The listing builds one solid part. Answer for the finished solid, in the listing's coordinates (mm). Face numbers are marked on the shaded views. A direction names the side the tool comes from. Round coordinates to 2 decimals unless told otherwise and drop trailing zeros. Loops run counter-clockwise (first coordinate to the right, second up) from the corner with the lowest first, then second, coordinate; pieces in that order, holes last. Notation, with made-up numbers: (76, 29) -> (134, 29) arc R7 cw to (134, 41) -> close; hole circle Ø10 at (30, -25). An arc over 180 degrees is marked (long way). Use a Markdown table: item, result. Add a question column.
Q1. Consider line 1 (Z direction, x = 2.25, y = 5.5) (3 decimals); line 2 (Z direction, x = 20, y = -4) (3 decimals); line 3 (Y direction, x = 1.75, z = 0). Determine where each line is inside the solid, lowest interval first.
Q2. Section B-B on y = 0 is taken. Give the vertices of the cut face in (x, z) (3 decimals), then the cut area to 3 significant figures.
Q3. Section D-D on x = 18.5 is taken. Give the vertices of the cut face in (y, z) (3 decimals).
Q4. Section C-C on z = 0 is taken. Give the vertices of the cut face in (x, y), then the cut area to 3 significant figures.
Q5. Which of the six approach directions +Z, -Z, +X, -X, +Y, -Y give full straight-line access (tool end or side, diameter ignored) to the marked faces 1 and 2?
Q6. Section A-A on x = 5.25 is taken. Give the vertices of the cut face in (y, z) (3 decimals).
Q7. Given pin 1 Ø8 at (y, z) = (7.5, -8) entering from +X; pin 2 Ø2.5 at (y, z) = (2.5, -21.5) entering from +X; pin 3 Ø1.8 at (x, y) = (12.84, 5.66) entering from +Z (3 decimals), each flat-ended and moving along its own axis, determine where each tip first touches the part or whether it passes through.
Q8. For a pull along Z with two mould halves and no side action, classify the marked faces 3, 4, 5 and 6 as released by +Z, released by -Z, zero draft, split by the parting line, or undercut.
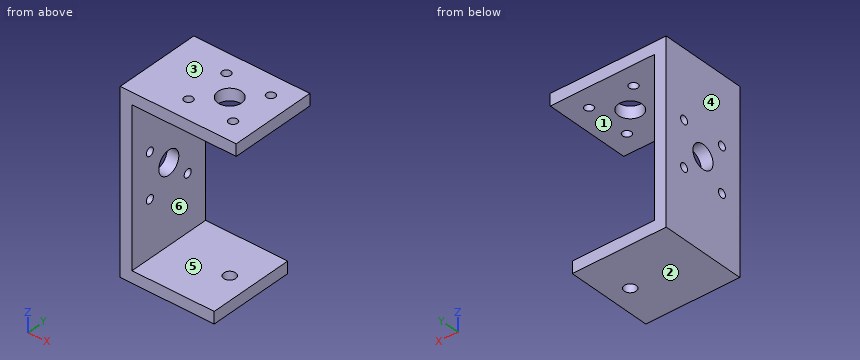
from build123d import *

# Parameters (mm, degrees)
SKETCH1_W           = 39.55
SKETCH1_H           = 22
SKETCH1_R           = 1.05
SKETCH1_R_2         = 3
BOSS_EXTRUDE1_DEPTH = 3
SKETCH1_6_W         = 3
SKETCH1_6_H         = 22
BOSS_EXTRUDE2_DEPTH = 29.5
SKETCH1_7_W         = 3
SKETCH1_7_H         = 22
BOSS_EXTRUDE3_DEPTH = 23.9
SKETCH2_R           = 3
SKETCH2_R_2         = 1.1
CUT_EXTRUDE1_DEPTH  = 3
CIRPATTERN1_COUNT   = 4
SKETCH3_R           = 1.5
CUT_EXTRUDE2_DEPTH  = 3


with BuildPart() as part:
    # Sketch1 → Boss-Extrude1 (new body)
    with BuildSketch(Plane(origin=(0, 0, 0), x_dir=(0, 0, -1), z_dir=(1, 0, 0))):
        Rectangle(SKETCH1_W, SKETCH1_H)
        with Locations((-5.656854249, -5.656854249)):
            Circle(SKETCH1_R, mode=Mode.SUBTRACT)
        with Locations((5.656854249, -5.656854249)):
            Circle(SKETCH1_R, mode=Mode.SUBTRACT)
        with Locations((-5.656854249, 5.656854249)):
            Circle(SKETCH1_R, mode=Mode.SUBTRACT)
        Circle(SKETCH1_R_2, mode=Mode.SUBTRACT)
        with Locations((5.656854249, 5.656854249)):
            Circle(SKETCH1_R, mode=Mode.SUBTRACT)
    extrude(amount=BOSS_EXTRUDE1_DEPTH)

    # Sketch1<6> → Boss-Extrude2 (add)
    with BuildSketch(Plane(origin=(0, 0, 0), x_dir=(0, 0, -1), z_dir=(1, 0, 0))):
        with Locations((-21.275, 0)):
            Rectangle(SKETCH1_6_W, SKETCH1_6_H)
    extrude(amount=BOSS_EXTRUDE2_DEPTH)

    # Sketch1<7> → Boss-Extrude3 (add)
    with BuildSketch(Plane(origin=(0, 0, 0), x_dir=(0, 0, -1), z_dir=(1, 0, 0))):
        with Locations((21.275, 0)):
            Rectangle(SKETCH1_7_W, SKETCH1_7_H)
    extrude(amount=BOSS_EXTRUDE3_DEPTH)

    # Sketch2 → Cut-Extrude1 (cut)
    with BuildSketch(Plane.XY.offset(22.775)):
        with Locations((18.5, 0)):
            Circle(SKETCH2_R)
        with Locations((24.156854249, 5.656854249)):
            Circle(SKETCH2_R_2)
    cut_extrude1 = extrude(amount=-CUT_EXTRUDE1_DEPTH, mode=Mode.SUBTRACT)

    # CirPattern1: Cut-Extrude1 ×4 about axis
    cirpattern1_axis = Axis((18.5, 0, 0), (0, 0, 1))
    for i in range(1, CIRPATTERN1_COUNT):
        add(cut_extrude1.rotate(cirpattern1_axis, i * 360 / CIRPATTERN1_COUNT), mode=Mode.SUBTRACT)

    # Sketch3 → Cut-Extrude2 (cut)
    with BuildSketch(Plane(origin=(0, 0, -22.775), x_dir=(-1, 0, 0), z_dir=(0, 0, -1))):
        with Locations((-18.5, 0)):
            Circle(SKETCH3_R)
    extrude(amount=-CUT_EXTRUDE2_DEPTH, mode=Mode.SUBTRACT)


solid = part.part
Checked values:
| question | item | result |
|---|---|---|
| 1 | line 1 | z = -22.775 to -6.695, -4.619 to 4.619, 6.695 to 22.775 |
| 1 | line 2 | z = -22.775 to -19.775, 19.775 to 22.775 |
| 1 | line 3 | y = -11 to -3, 3 to 11 |
| 2 | outline | (0, -22.775) -> (17, -22.775) -> (17, -19.775) -> (3, -19.775) -> (3, -3) -> (0, -3) -> close; (0, 3) -> (3, 3) -> (3, 19.775) -> (15.5, 19.775) -> (15.5, 22.775) -> (0, 22.775) -> close; (20, -22.775) -> (23.9, -22.775) -> (23.9, -19.775) -> (20, -19.775) -> close; (21.5, 19.775) -> (29.5, 19.775) -> (29.5, 22.775) -> (21.5, 22.775) -> close |
| 2 | area | 234 mm2 |
| 3 | outline | (-11, -22.775) -> (-1.5, -22.775) -> (-1.5, -19.775) -> (-11, -19.775) -> close; (-11, 19.775) -> (-3, 19.775) -> (-3, 22.775) -> (-11, 22.775) -> close; (1.5, -22.775) -> (11, -22.775) -> (11, -19.775) -> (1.5, -19.775) -> close; (3, 19.775) -> (11, 19.775) -> (11, 22.775) -> (3, 22.775) -> close |
| 4 | outline | (0, -11) -> (3, -11) -> (3, -3) -> (0, -3) -> close; (0, 3) -> (3, 3) -> (3, 11) -> (0, 11) -> close |
| 4 | area | 48.0 mm2 |
| 5 | face 1 | +X, +Y, -Y |
| 5 | face 2 | -Z, +X, -X, +Y, -Y |
| 6 | outline | (-11, -22.775) -> (11, -22.775) -> (11, -19.775) -> (-11, -19.775) -> close; (-11, 19.775) -> (11, 19.775) -> (11, 22.775) -> (-11, 22.775) -> close |
| 7 | pin 1 | stops at x = 3 |
| 7 | pin 2 | stops at x = 23.9 |
| 7 | pin 3 | stops at z = -19.775 |
| 8 | face 3 | released by +Z |
| 8 | face 4 | zero draft |
| 8 | face 5 | undercut |
| 8 | face 6 | undercut |
